The listing builds one solid part. Answer for the finished solid, in the listing's coordinates (mm). Face numbers are marked on the shaded views. A direction names the side the tool comes from. Coordinates: 2 decimals unless noted, no trailing zeros. Loops run counter-clockwise (first coordinate to the right, second up) from the corner with the lowest first, then second, coordinate; pieces in that order, holes last. Notation, with made-up numbers: (59.5, -23.5) - (77.5, -23.5) arc R19 cw to (77.5, -16.5) - close; hole circle Ø8 at (60.25, 40). An arc over 180 degrees is marked (long way). Return JSON: item names as keys, results as strings. Group by question number.
1. Section A-A (y = 34) is taken. Write down the section's boundary in (x, z), and give its area (3 significant figures).
2. Each of these flat-tipped pins is pushed along its axis until it touches: P1, Ø10, axis at x = 27, z = 21.5, coming from the +Y side; P2, Ø2.5, axis at y = 34, z = 24, coming from the -X side; P3, Ø1.2, axis at x = 18.5, z = 24, coming from the -Y side; P4, Ø12.5, axis at y = 33.5, z = 20.5, coming from the -X side. Where does it stop, or does it pass through?
3. Find the intervals of material crossed by line 1 along Y through (x, z) = (4.45, 24); line 2 along X through (y, z) = (-2, 17.5); line 3 along Y through (x, z) = (8, 22.25), in increasing order.
4. Section C-C (z = 24) is taken. Write down the section's boundary in (x, y), and give its area (3 significant figures).
5. Section B-B (x = 3) is taken. Write down the section's boundary in (y, z), and give its area (3 significant figures).
6. Section D-D (x = 19) is taken. Write down the section's boundary in (y, z), and give its area (3 significant figures).
7. Which of the six approach directions +Z, -Z, +X, -X, +Y, -Y give full straight-line access (tool end or side, diameter ignored) to the marked faces 1, 2 and 3?
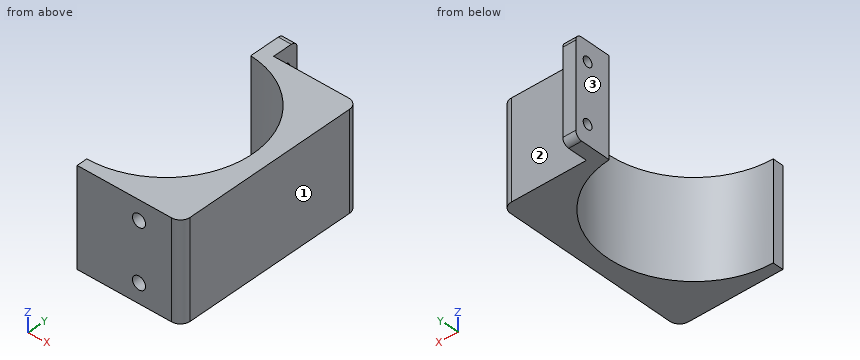
```python
from build123d import *

# Parameters (mm, degrees)
EXTRUDE_1_DEPTH     = 30
FILLET_1_R          = 3
SKETCH_3_R          = 2
CUT_EXTRUDE_1_DEPTH = 7
SKETCH_4_R          = 1.5
CUT_EXTRUDE_2_DEPTH = 62.546730214
SKETCH_5_W          = 141.789042775
SKETCH_5_H          = 177.448562515
CUT_EXTRUDE_3_DEPTH = 59.034472514
FILLET_2_R          = 2


with BuildPart() as part:
    # 草图1 → 凸台-拉伸1 (new body)
    with BuildSketch(Plane.XY):
        with BuildLine():
            Line((-32, 30), (-6, 30))
            Line((-6, 30), (-6, 38))
            Line((-6, 38), (-2, 38))
            Line((-2, 38), (-2, 28.659348025))
            Line((-2, 28.659348025), (-2, 26.675128866))
            ThreePointArc((-2, 26.675128866), (0, -26.75), (2, 26.675128866))
            Line((2, 26.675128866), (2, 28.659348025))
            Line((2, 28.659348025), (2, 38))
            Line((2, 38), (6, 38))
            Line((6, 38), (6, 30))
            Line((6, 30), (32, 30))
            Line((32, 30), (32, -30))
            Line((32, -30), (-32, -30))
            Line((-32, -30), (-32, 30))
        make_face()
    extrude(amount=EXTRUDE_1_DEPTH)

    # 圆角1
    fillet_1_edges = [part.edges().sort_by_distance(p)[0] for p in [
        (32, -30, 15),
        (-32, -30, 15),
        (-32, 30, 15),
        (32, 30, 15),
    ]]
    fillet(fillet_1_edges, radius=FILLET_1_R)

    # 草图3 → 切除-拉伸1 (cut)
    with BuildSketch(Plane.XZ.offset(30)):
        with Locations(Location((19, 24, 0), (0, 0, 270))):
            Circle(SKETCH_3_R)
        with Locations(Location((19, 6, 0), (0, 0, 270))):
            Circle(SKETCH_3_R)
    extrude(amount=-CUT_EXTRUDE_1_DEPTH, mode=Mode.SUBTRACT)

    # 草图4 → 切除-拉伸2 (cut, through all)
    with BuildSketch(Plane(origin=(6, 0, 0), x_dir=(0, 0, -1), z_dir=(1, 0, 0))):
        with Locations((-24, 34)):
            Circle(SKETCH_4_R)
        with Locations((-6, 34)):
            Circle(SKETCH_4_R)
    extrude(amount=-CUT_EXTRUDE_2_DEPTH, mode=Mode.SUBTRACT)

    # 草图5 → 切除-拉伸3 (cut, through all)
    with BuildSketch(Plane(origin=(0, 0, 0), x_dir=(0, 0, -1), z_dir=(1, 0, 0))):
        with Locations((-47.884475127, 49.870130309)):
            Rectangle(SKETCH_5_W, SKETCH_5_H)
    extrude(amount=-CUT_EXTRUDE_3_DEPTH, mode=Mode.SUBTRACT)

    # 圆角2
    fillet_2_edges = [part.edges().sort_by_distance(p)[0] for p in [
        (4, 38, 30),
        (4, 38, 0),
    ]]
    fillet(fillet_2_edges, radius=FILLET_2_R)


solid = part.part
```
The answers:
{
 "1": {"outline": "(2, 0) - (6, 0) - (6, 4.5) - (2, 4.5) - close; (2, 7.5) - (6, 7.5) - (6, 22.5) - (2, 22.5) - close; (2, 25.5) - (6, 25.5) - (6, 30) - (2, 30) - close", "area": "96.0 mm2"},
 "2": {"P1": "stops at y = 30", "P2": "passes through", "P3": "stops at y = -23", "P4": "stops at x = 2"},
 "3": {"line 1": "y = -30 to -26.38, 26.38 to 32.5, 35.5 to 38", "line 2": "x = 26.68 to 32", "line 3": "y = -30 to -25.53, 25.53 to 30"},
 "4": {"outline": "(0, -30) - (17, -30) - (17, -23) - (21, -23) - (21, -30) - (29, -30) arc R3 ccw to (32, -27) - (32, 27) arc R3 ccw to (29, 30) - (6, 30) - (6, 32.5) - (2, 32.5) - (2, 26.68) arc R26.75 cw to (0, -26.75) - close; (2, 35.5) - (6, 35.5) - (6, 38) - (2, 38) - close", "area": "778 mm2"},
 "5": {"outline": "(-30, 0) - (-26.58, 0) - (-26.58, 30) - (-30, 30) - close; (26.58, 0) - (36, 0) arc R2 ccw to (38, 2) - (38, 28) arc R2 ccw to (36, 30) - (26.58, 30) - close; hole circle Ø3 at (34, 6); hole circle Ø3 at (34, 24)", "area": "429 mm2"},
 "6": {"outline": "(-30, 0) - (-18.83, 0) - (-18.83, 30) - (-30, 30) - (-30, 26) - (-23, 26) - (-23, 22) - (-30, 22) - (-30, 8) - (-23, 8) - (-23, 4) - (-30, 4) - close; (18.83, 0) - (30, 0) - (30, 30) - (18.83, 30) - close", "area": "614 mm2"},
 "7": {"face 1": "+Z, -Z, +X, +Y, -Y", "face 2": "+Z, -Z, +X, +Y", "face 3": "+Z, -Z, -X, +Y"}
}
